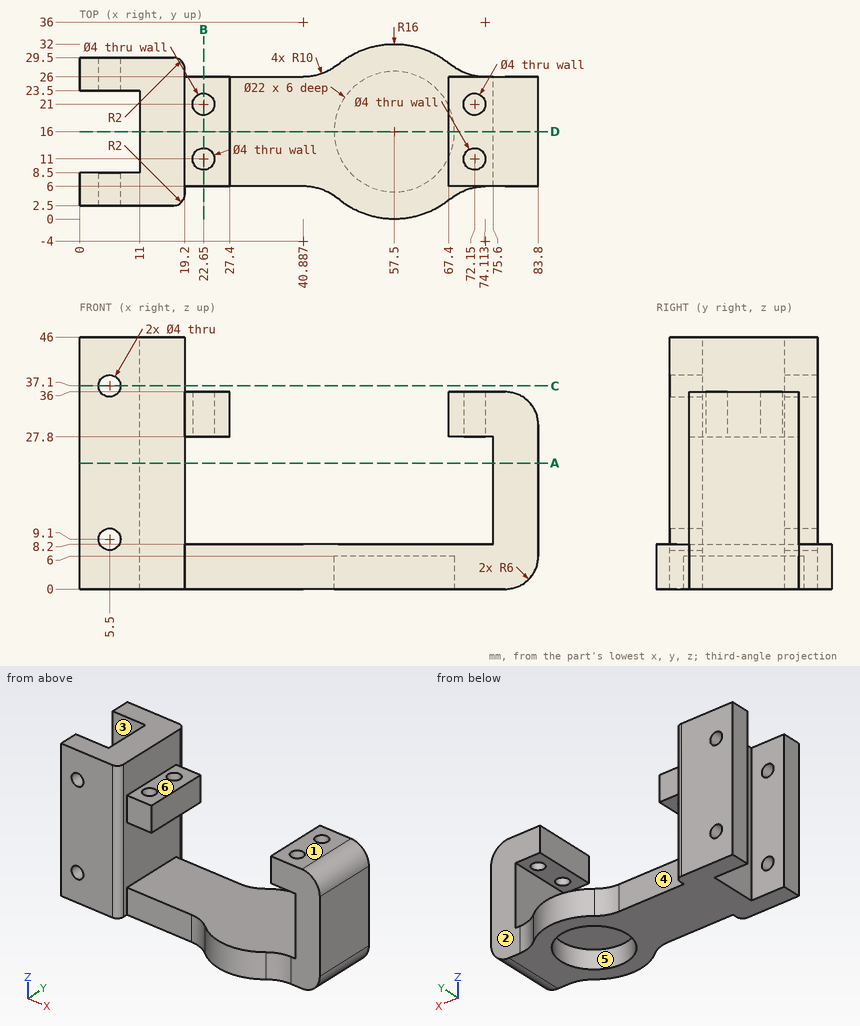
Study the drawing (mm; zero at the part's minimum x, y, z) and answer. A direction names the side the tool comes from. Coordinates: 2 decimals unless noted, no trailing zeros. Loops run counter-clockwise (first coordinate to the right, second up) from the corner with the lowest first, then second, coordinate; pieces in that order, holes last. Notation, with made-up numbers: M 69.25,6 L 116.25,6 A30 cw 116.25,38 Z; hole C -18,64.5 d5. An arc over 180 degrees is marked long. Answer in a Markdown table with one row per item. Add a question column.
1. Flat-ended cylindrical pins translate along their axes: P1, Ø12, axis at x = 52, y = 13, coming from the +Z side; P2, Ø5, axis at x = 5.5, z = 9.1, coming from the -Y side; P3, Ø12, axis at y = 18, z = 30.5, coming from the -X side; P4, Ø4, axis at x = 22.5, z = 30.5, coming from the -Y side. Find the tip coordinate at first contact, or state that the pin passes through.
2. Find section D-D, the plane y = 16. Write down the section's boundary in (x, z), then the cut area to 3 significant figures.
3. Consider L1, parallel to Z at x = 5.5, y = 4.8; L2, parallel to Z at x = 69, y = 11.5; L3, parallel to X at y = 13, z = 11.5. Determine where each line is inside the solid, lowest interval first.
4. The mould has two halves that part along Y. Classify the marked faces 1, 2 and 3: pulls with the +Y half, pulls with the -Y half, needs draft (parallel to the pull), parting line crosses it, or undercut.
5. Find section B-B, the plane x = 22.65. Write down the section's boundary in (y, z), then the cut area to 3 significant figures.
6. A tool of negligible diameter and unlimited length cuts with its end or side. For the marked faces 4, 5 and 6, from which of +Z, -Z, +X, -X, +Y, -Y can it reach the whole face along a straight path? Write none if from no direction.
7. Find section A-A, the plane z = 23. Write down the section's boundary in (x, y), then the cut area to 3 significant figures.
8. Find section C-C, the plane z = 37.1. Write down the section's boundary in (x, y).
Reported:
| question | item | result |
|---|---|---|
| 1 | P1 | stops at z = 8.2 |
| 1 | P2 | stops at y = 2.5 |
| 1 | P3 | stops at x = 0 |
| 1 | P4 | stops at y = 6 |
| 2 | outline | M 11,0 L 46.5,0 L 46.5,6 L 68.5,6 L 68.5,0 L 77.8,0 A6 ccw 83.8,6 L 83.8,30 A6 ccw 77.8,36 L 67.4,36 L 67.4,27.8 L 75.6,27.8 L 75.6,8.2 L 19.2,8.2 L 19.2,27.8 L 27.4,27.8 L 27.4,36 L 19.2,36 L 19.2,46 L 11,46 Z |
| 2 | area | 1,120 mm^2 |
| 3 | L1 | z = 0 to 7.1, 11.1 to 35.1, 39.1 to 46 |
| 3 | L2 | z = 0 to 8.2, 27.8 to 36 |
| 3 | L3 | x = 11 to 19.2, 75.6 to 83.8 |
| 4 | face 1 | needs draft |
| 4 | face 2 | pulls with the +Y half |
| 4 | face 3 | undercut |
| 5 | outline | M 6,0 L 26,0 L 26,8.2 L 6,8.2 Z; M 6,27.8 L 9,27.8 L 9,36 L 6,36 Z; M 13,27.8 L 19,27.8 L 19,36 L 13,36 Z; M 23,27.8 L 26,27.8 L 26,36 L 23,36 Z |
| 5 | area | 262 mm^2 |
| 6 | face 4 | +Z, -Z, +Y |
| 6 | face 5 | -Z |
| 6 | face 6 | +Z, +X, +Y, -Y |
| 7 | outline | M 0,2.5 L 17.2,2.5 A2 ccw 19.2,4.5 L 19.2,27.5 A2 ccw 17.2,29.5 L 0,29.5 L 0,23.5 L 11,23.5 L 11,8.5 L 0,8.5 Z; M 75.6,6 L 83.8,6 L 83.8,26 L 75.6,26 Z |
| 7 | area | 516 mm^2 |
| 8 | outline | M 0,2.5 L 3.5,2.5 L 3.5,8.5 L 0,8.5 Z; M 0,23.5 L 3.5,23.5 L 3.5,29.5 L 0,29.5 Z; M 7.5,2.5 L 17.2,2.5 A2 ccw 19.2,4.5 L 19.2,27.5 A2 ccw 17.2,29.5 L 7.5,29.5 L 7.5,23.5 L 11,23.5 L 11,8.5 L 7.5,8.5 Z |
